Can you work these out from the model? Positions are in its coordinate system, mm. Face numbers are marked on the shaded views. A direction names the side the tool comes from. Round coordinates to 2 decimals unless told otherwise and drop trailing zeros. Write each loop counter-clockwise with the first axis right and the second up, starting at its lowest first coordinate (ties: lowest second). Pieces come first, ordered by that corner, then holes.
Q1. If we section it at A-A (z = 29): Please give me the cut outline in (x, y), plus the area to 3 significant figures.
Q2. If we section it at B-B (y = 3): Please give me the cut outline in (x, z).
Q3. If we section it at D-D (x = 40): Please give me the cut outline in (y, z).
Q4. If we section it at C-C (x = 20.5): Please give me the cut outline in (y, z).
Q5. I'm going to push flat-ended pins straight in: pin 1 Ø12 at (y, z) = (8.5, 24.5) entering from -X; pin 2 Ø2.5 at (y, z) = (1, 2) entering from +X. Where does each tip first touch, or does it pass through?
Q6. Please list where these lines run through material, in increasing order: line 1 along Z through (x, y) = (62.1, 0); line 2 along Y through (x, z) = (40, 2.6); line 3 along Z through (x, y) = (61, 0).
Q7. For the marked faces 1 and 2, which set-ups out of +Z, -Z, +X, -X, +Y, -Y let a thin tool reach every point of the face, with its end or its side?
from build123d import *

# Parameters (mm, degrees)
SKETCH_W     = 75
SKETCH_H     = 30
SKETCH_R     = 1.75
SKETCH_W_2   = 15
SKETCH_H_2   = 20
PAD_DEPTH    = 5
FILLET_R     = 10
FILLET001_R  = 1
SKETCH001_W  = 5
SKETCH001_H  = 30
PAD001_DEPTH = 30
FILLET002_R  = 5
FILLET003_R  = 5
SKETCH002_R  = 2.25
POCKET_DEPTH = 75.001
CHAMFER_SIZE = 10


with BuildPart() as part:
    # Sketch → Pad (new body)
    with BuildSketch(Plane.XY):
        with Locations((27.5, 0)):
            Rectangle(SKETCH_W, SKETCH_H)
        Circle(SKETCH_R, mode=Mode.SUBTRACT)
        with Locations((40, 0)):
            Circle(SKETCH_R, mode=Mode.SUBTRACT)
        with Locations((20, 0)):
            Rectangle(SKETCH_W_2, SKETCH_H_2, mode=Mode.SUBTRACT)
    extrude(amount=PAD_DEPTH)

    # Fillet
    fillet_edges = [part.edges().sort_by_distance(p)[0] for p in [
        (-10, 15, 2.5),
        (-10, -15, 2.5),
    ]]
    fillet(fillet_edges, radius=FILLET_R)

    # Fillet001
    fillet001_edges = [part.edges().sort_by_distance(p)[0] for p in [
        (12.5, 0, 5),
        (12.5, 0, 0),
        (20, 10, 0),
        (20, 10, 5),
        (27.5, 0, 5),
        (20, -10, 5),
        (27.5, 0, 0),
        (20, -10, 0),
    ]]
    fillet(fillet001_edges, radius=FILLET001_R)

    # Sketch001 (on Face18 of Fillet001) → Pad001 (join)
    with BuildSketch(Plane.XY.offset(5)):
        with Locations((62.5, 0)):
            Rectangle(SKETCH001_W, SKETCH001_H)
    extrude(amount=PAD001_DEPTH)

    # Fillet002
    fillet002_edges = [part.edges().sort_by_distance(p)[0] for p in [
        (65, 0, 0),
    ]]
    fillet(fillet002_edges, radius=FILLET002_R)

    # Fillet003
    fillet003_edges = [part.edges().sort_by_distance(p)[0] for p in [
        (60, 0, 5),
    ]]
    fillet(fillet003_edges, radius=FILLET003_R)

    # Sketch002 (on Face9 of Fillet003) → Pocket (cut, through all)
    with BuildSketch(Plane.YZ.offset(65)):
        with Locations((0, 29)):
            Circle(SKETCH002_R)
        with Locations((0, 14)):
            Circle(SKETCH002_R)
    extrude(amount=-POCKET_DEPTH, mode=Mode.SUBTRACT)

    # Chamfer
    chamfer_edges = [part.edges().sort_by_distance(p)[0] for p in [
        (62.5, -15, 35),
        (62.5, 15, 35),
    ]]
    chamfer(chamfer_edges, length=CHAMFER_SIZE)


solid = part.part
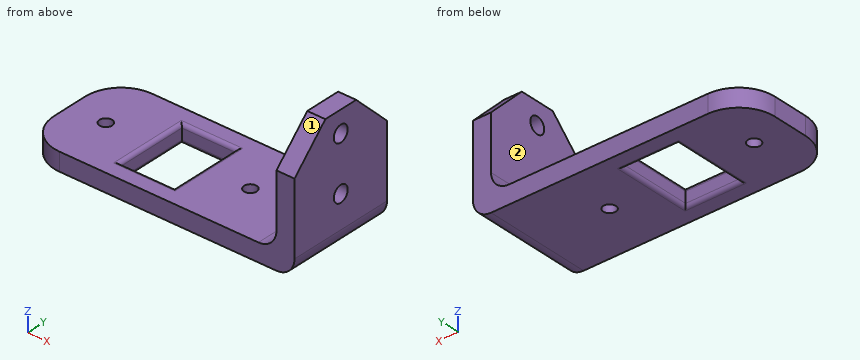
A:
1. outline: (60, -11) - (65, -11) - (65, -2.25) - (60, -2.25) - close; (60, 2.25) - (65, 2.25) - (65, 11) - (60, 11) - close
1. area: 87.5 mm2
2. outline: (-10, 0) - (11.5, 0) arc R1 ccw to (12.5, 1) - (12.5, 4) arc R1 ccw to (11.5, 5) - (-10, 5) - close; (27.5, 1) arc R1 ccw to (28.5, 0) - (60, 0) arc R5 ccw to (65, 5) - (65, 35) - (60, 35) - (60, 10) arc R5 cw to (55, 5) - (28.5, 5) arc R1 ccw to (27.5, 4) - close
3. outline: (-15, 0) - (-1.75, 0) - (-1.75, 5) - (-15, 5) - close; (1.75, 0) - (15, 0) - (15, 5) - (1.75, 5) - close
4. outline: (-15, 0) - (-11, 0) arc R1 ccw to (-10, 1) - (-10, 4) arc R1 ccw to (-11, 5) - (-15, 5) - close; (10, 1) arc R1 ccw to (11, 0) - (15, 0) - (15, 5) - (11, 5) arc R1 ccw to (10, 4) - close
5. pin 1: stops at x = 60
5. pin 2: stops at x = 64.68
6. line 1: z = 0.46 to 11.75, 16.25 to 26.75, 31.25 to 35
6. line 2: y = -15 to -1.75, 1.75 to 15
6. line 3: z = 0.1 to 11.75, 16.25 to 26.75, 31.25 to 35
7. face 1: +Z, +X, -X, -Y
7. face 2: +Z, -X, +Y, -Y
